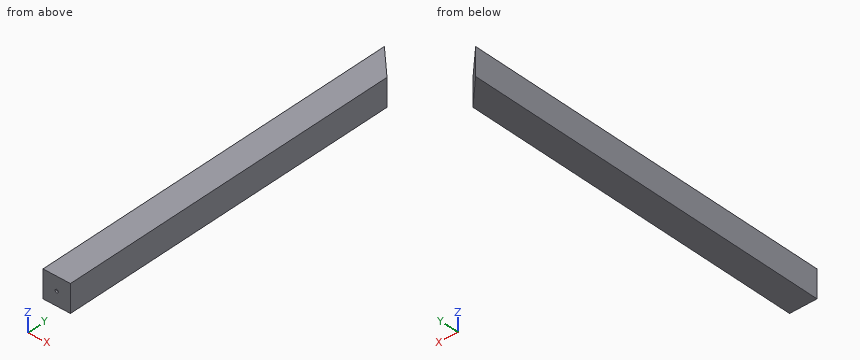
from build123d import *

# Parameters (mm, degrees)
SKETCH1_W               = 25.4
SKETCH1_H               = 25.4
BOSS_EXTRUDE1_DEPTH     = 174.485
CUT_EXTRUDE1_DEPTH      = 13.7
CUT_EXTRUDE1_DEPTH_BACK = 13.7


with BuildPart() as part:
    # Sketch1 → Boss-Extrude1 (new body, symmetric)
    with BuildSketch(Plane(origin=(0, 0, 0), x_dir=(1, 0, 0), z_dir=(0, 1, 0))):
        Rectangle(SKETCH1_W, SKETCH1_H)
    extrude(amount=BOSS_EXTRUDE1_DEPTH, both=True)

    # Sketch3 → #0-80 Tapped Hole1 (revolve, cut)
    with BuildSketch(Plane(origin=(0, -174.485, 0), x_dir=(0, 0, -1), z_dir=(1, 0, 0))):
        Polygon((0, 0), (0, 20.357890611), (0.59563, 20), (0.59563, 0.768338359), (1.5113, 0), align=None)
    f_0_80_tapped_hole1 = revolve(axis=Axis((0, -180.835, 0), (0, 1, 0)), mode=Mode.SUBTRACT)

    # Mirror1: #0-80 Tapped Hole1 across plane
    add(f_0_80_tapped_hole1.mirror(Plane.ZX), mode=Mode.SUBTRACT)

    # Sketch4 → Cut-Extrude1 (cut, two sides)
    with BuildSketch(Plane.XY) as cut_extrude1_sk:
        Polygon((12.7, 174.485), (-12.7, 174.485), (12.7, 149.085), align=None)
    extrude(amount=CUT_EXTRUDE1_DEPTH, mode=Mode.SUBTRACT)
    extrude(cut_extrude1_sk.sketch, amount=-CUT_EXTRUDE1_DEPTH_BACK, mode=Mode.SUBTRACT)


solid = part.part
Could you check a few things on this model? Use its own coordinates, in mm. Coordinates: 2 decimals unless noted, no trailing zeros. Loops run counter-clockwise (first coordinate to the right, second up) from the corner with the lowest first, then second, coordinate; pieces in that order, holes last.
1. I need wall thicknesses on L1, parallel to Z at x = 0, y = -158.25; L2, parallel to Y at x = 0.5, z = 2.75 (3 decimals). Which ranges of each line are inside material? Lowest first, please.
2. Imagine slicing it at A-A (z = 6.5). Please give me the cut outline in (x, y) (3 decimals).
3. For P1, Ø1.5, axis at x = 0, z = 0, coming from the -Y side; P2, Ø0.7, axis at x = 0, z = 0, coming from the +Y side, each with a flat end and sliding along its axis, tell me the tip position at first contact or that it passes through.
Computed values:
1. L1: z = -12.7 to -0.6, 0.6 to 12.7
1. L2: y = -174.485 to 161.285
2. outline: (-12.7, -174.485) - (12.7, -174.485) - (12.7, 149.085) - (-12.7, 174.485) - close
3. P1: stops at y = -173.85
3. P2: stops at y = 154.34
